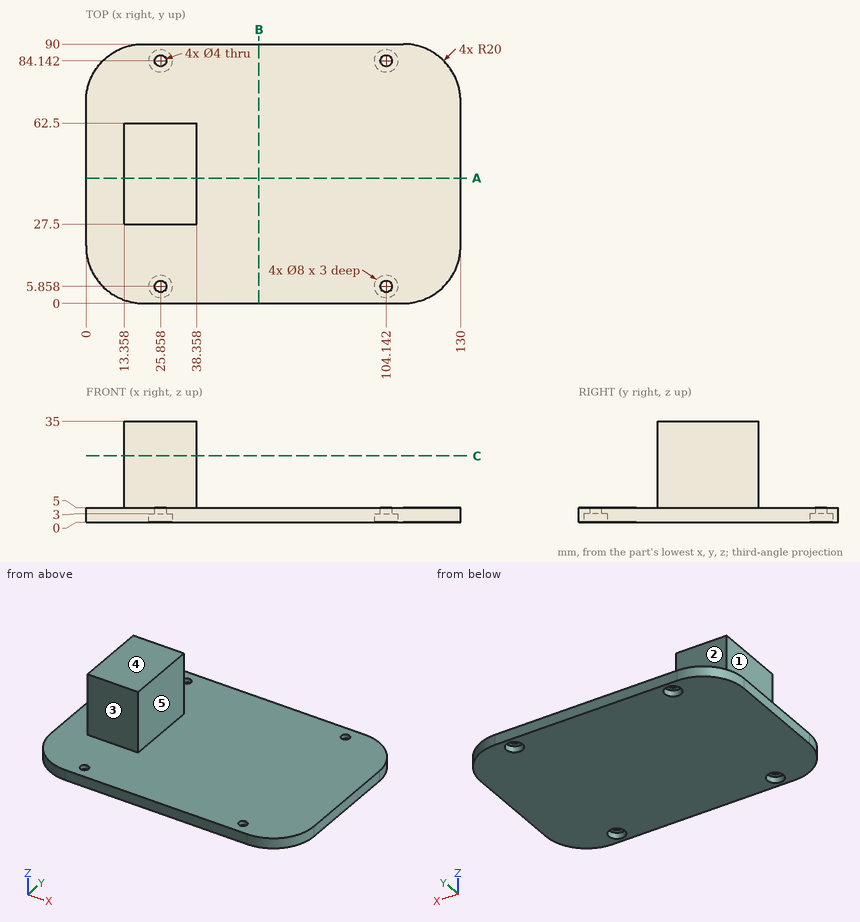
Print and shaded views of the part. All mm, measured from the part's lowest x, y and z. A direction names the side the tool comes from. Coordinates: 2 decimals unless noted, no trailing zeros. Write each loop counter-clockwise with the first axis right and the second up, starting at its lowest first coordinate (ties: lowest second). Pieces come first, ordered by that corner, then holes.
(1) Flat gauge pins, fed straight in: pin 1 (4 mm diameter, centred on x = 54, y = 43.5, fed in from -Z); pin 2 (12 mm diameter, centred on x = 66, y = 40.5, fed in from +Z); pin 3 (20 mm diameter, centred on x = 27, z = 22.5, fed in from +Y); pin 4 (2.5 mm diameter, centred on x = 104.14, y = 84.14, fed in from -Z). Where does each tip first touch, or does it go through?
(2) Cut at A-A, the plane y = 43.5. List the corners of the cut face in (x, z), and give its area (3 significant figures).
(3) Drill centre lines: probe 1 along Z at (x, y) = (10.5, 47); probe 2 along X at (y, z) = (39, 7.5); probe 3 along Y at (x, z) = (23, 17.5). Where is each one in solid material? Low to high.
(4) Cut at C-C, the plane z = 23. List the corners of the cut face in (x, y), and give its area (3 significant figures).
(5) Cut at B-B, the plane x = 60. List the corners of the cut face in (y, z), and give its area (3 significant figures).
(6) 3-axis set-ups, long thin cutter, end or side, ignore diameter. For the marked faces 1, 2, 3, 4 and 5: which of +Z, -Z, +X, -X, +Y, -Y reach the whole face in a straight line?
Geometry says:
1. pin 1: stops at z = 0
1. pin 2: stops at z = 5
1. pin 3: stops at y = 62.5
1. pin 4: passes through
2. outline: (0, 0) - (130, 0) - (130, 5) - (38.36, 5) - (38.36, 35) - (13.36, 35) - (13.36, 5) - (0, 5) - close
2. area: 1,400 mm2
3. probe 1: z = 0 to 5
3. probe 2: x = 13.36 to 38.36
3. probe 3: y = 27.5 to 62.5
4. outline: (13.36, 27.5) - (38.36, 27.5) - (38.36, 62.5) - (13.36, 62.5) - close
4. area: 875 mm2
5. outline: (0, 0) - (90, 0) - (90, 5) - (0, 5) - close
5. area: 450 mm2
6. face 1: +Z, -X, +Y, -Y
6. face 2: +Z, +X, -X, +Y
6. face 3: +Z, +X, -X, -Y
6. face 4: +Z, +X, -X, +Y, -Y
6. face 5: +Z, +X, +Y, -Y
